Part model, mm, in its own coordinate system. Coordinates: 2 decimals unless noted, no trailing zeros. Order: outer loops, then holes, each group sorted by start corner. A loop starts at its lowest first (then second) coordinate and runs counter-clockwise, first axis right, second up.
1) Pin check, flat tips, straight feed: pin 1 Ø12 at (x, z) = (-60.5, 86) entering from -Y; pin 2 Ø6 at (y, z) = (-39.5, 130.5) entering from -X; pin 3 Ø1.5 at (y, z) = (-13.5, 134) entering from -X; pin 4 Ø10 at (x, z) = (-67.5, 26.5) entering from -Y. Stop position of each tip, or through.
2) Cut at C-C (y = -93.5). List the corners of the cut face in (x, z).
3) Cut at B-B (x = 14). List the corners of the cut face in (y, z), and give its area (3 significant figures).
4) Wall check: L1, parallel to Y at x = 12.5, z = 67; L2, parallel to Z at x = 67, y = -35; L3, parallel to X at y = -48, z = 54.5. Give the ranges that are in metal, low to high.
5) Cut at A-A (z = 69). List the corners of the cut face in (x, y).
```python
from build123d import *

# Parameters (mm, degrees)
BOSS_EXTRU_1_DEPTH            = 170
ENL_V_MAT_EXTRU_1_DEPTH       = 220
ENL_V_MAT_EXTRU_2_DEPTH       = 220
ENL_V_MAT_EXTRU_3_DEPTH       = 220
ENL_V_MAT_EXTRU_4_DEPTH       = 220
ENL_V_MAT_EXTRU_11_DEPTH      = 220
ENL_V_MAT_EXTRU_13_DEPTH      = 220
ENL_V_MAT_EXTRU_13_DEPTH_BACK = 220
ENL_V_MAT_EXTRU_14_DEPTH      = 220
ENL_V_MAT_EXTRU_15_DEPTH      = 220
ENL_V_MAT_EXTRU_15_DEPTH_BACK = 220
ENL_V_MAT_EXTRU_16_DEPTH      = 220
ENL_V_MAT_EXTRU_17_DEPTH      = 220
ENL_V_MAT_EXTRU_17_DEPTH_BACK = 220
ENL_V_MAT_EXTRU_18_DEPTH      = 220
ENL_V_MAT_EXTRU_19_DEPTH      = 220
ENL_V_MAT_EXTRU_19_DEPTH_BACK = 220
ENL_V_MAT_EXTRU_20_DEPTH      = 220
ENL_V_MAT_EXTRU_20_DEPTH_BACK = 220
ENL_V_MAT_EXTRU_21_DEPTH      = 220
ENL_V_MAT_EXTRU_21_DEPTH_BACK = 220
ENL_V_MAT_EXTRU_22_DEPTH      = 220
ENL_V_MAT_EXTRU_22_DEPTH_BACK = 220
ENL_V_MAT_EXTRU_23_DEPTH      = 220
ENL_V_MAT_EXTRU_23_DEPTH_BACK = 220
CONG_2_R                      = 15
ESQUISSE26_R                  = 11.42194069
BOSS_EXTRU_2_DEPTH            = 30
CONG_6_R                      = 10


with BuildPart() as part:
    # Esquisse1 → Boss.-Extru.1 (new body)
    with BuildSketch(Plane.XY):
        Polygon((-32, 85), (32, 85), (85, 32), (85, -32), (32, -85), (-32, -85), (-85, -32), (-85, 32), align=None)
    extrude(amount=BOSS_EXTRU_1_DEPTH)

    # Esquisse3D3 → Enlèv. mat.-Extru.1 (cut, along a direction that is not the sketch's normal)
    with BuildSketch(Plane(origin=(-32, 85, 117), x_dir=(0.6493531093113899, -0.5377455436484948, 0.5377455436484945), z_dir=(0, 0.7071067811865474, 0.7071067811865478))):
        Polygon((0, 0), (57.001027627, -48.67117062), (98.559626623, 0), (41.558598996, 48.67117062), align=None)
    extrude(amount=ENL_V_MAT_EXTRU_1_DEPTH, dir=(0, 0, 1), mode=Mode.SUBTRACT)

    # Esquisse3D4 → Enlèv. mat.-Extru.2 (cut, along a direction that is not the sketch's normal)
    with BuildSketch(Plane(origin=(32, 85, 53), x_dir=(-0.6493531093113893, -0.537745543648495, -0.537745543648495), z_dir=(0, -0.7071067811865476, 0.7071067811865476))):
        Polygon((0, 0), (57.001027627, 48.67117062), (98.559626623, 0), (41.558598996, -48.67117062), align=None)
    extrude(amount=-ENL_V_MAT_EXTRU_2_DEPTH, dir=(0, 0, 1), mode=Mode.SUBTRACT)

    # Esquisse3D5 → Enlèv. mat.-Extru.3 (cut, along a direction that is not the sketch's normal)
    with BuildSketch(Plane(origin=(-32, -85, 53), x_dir=(0.6493531093113899, 0.5377455436484946, -0.5377455436484948), z_dir=(0, 0.7071067811865479, 0.7071067811865472))):
        Polygon((0, 0), (57.001027627, 48.67117062), (98.559626623, 0), (41.558598996, -48.67117062), align=None)
    extrude(amount=-ENL_V_MAT_EXTRU_3_DEPTH, dir=(0, 0, 1), mode=Mode.SUBTRACT)

    # Esquisse3D6 → Enlèv. mat.-Extru.4 (cut, along a direction that is not the sketch's normal)
    with BuildSketch(Plane(origin=(32, -85, 117), x_dir=(-0.6493531093113899, 0.5377455436484946, 0.5377455436484947), z_dir=(0, 0.7071067811865476, -0.7071067811865476))):
        Polygon((0, 0), (57.001027627, 48.67117062), (98.559626623, 0), (41.558598996, -48.67117062), align=None)
    extrude(amount=-ENL_V_MAT_EXTRU_4_DEPTH, dir=(0, 0, -1), mode=Mode.SUBTRACT)

    # Esquisse3D13 → Enlèv. mat.-Extru.11 (cut, along a direction that is not the sketch's normal)
    with BuildSketch(Plane(origin=(32, 32, 170), x_dir=(0.5377455436484943, -0.6493531093113897, -0.5377455436484953), z_dir=(-0.7071067811865481, 0, -0.7071067811865469))):
        Polygon((0, 0), (57.001027627, -48.67117062), (98.559626623, 0), (41.558598996, 48.67117062), align=None)
    extrude(amount=-ENL_V_MAT_EXTRU_11_DEPTH, dir=(-1, 0, 0), mode=Mode.SUBTRACT)

    # Esquisse16 → Enlèv. mat.-Extru.13 (cut, two sides: drawn at the far end of the back side and taken through both)
    with BuildSketch(Plane(origin=(0, -32, 0), x_dir=(1, 0, 0), z_dir=(0, 1, 0)).offset(-ENL_V_MAT_EXTRU_13_DEPTH_BACK)):
        Polygon((32, -170), (85, -170), (85, -117), align=None)
    extrude(amount=ENL_V_MAT_EXTRU_13_DEPTH + ENL_V_MAT_EXTRU_13_DEPTH_BACK, mode=Mode.SUBTRACT)

    # Esquisse3D15 → Enlèv. mat.-Extru.14 (cut, along a direction that is not the sketch's normal)
    with BuildSketch(Plane(origin=(-85, -32, 117), x_dir=(0.5377455436484945, 0.6493531093113897, 0.5377455436484953), z_dir=(0.707106781186548, 0, -0.707106781186547))):
        Polygon((0, 0), (57.001027627, 48.67117062), (98.559626623, 0), (41.558598996, -48.67117062), align=None)
    extrude(amount=-ENL_V_MAT_EXTRU_14_DEPTH, dir=(0, 0, -1), mode=Mode.SUBTRACT)

    # Esquisse17 → Enlèv. mat.-Extru.15 (cut, two sides: drawn at the far end of the back side and taken through both)
    with BuildSketch(Plane(origin=(0, -32, 0), x_dir=(1, 0, 0), z_dir=(0, 1, 0)).offset(-ENL_V_MAT_EXTRU_15_DEPTH_BACK)):
        Polygon((-85, -117), (-32, -170), (-85, -170), align=None)
    extrude(amount=ENL_V_MAT_EXTRU_15_DEPTH + ENL_V_MAT_EXTRU_15_DEPTH_BACK, mode=Mode.SUBTRACT)

    # Esquisse3D16 → Enlèv. mat.-Extru.16 (cut, along a direction that is not the sketch's normal)
    with BuildSketch(Plane(origin=(-32, 32, 0), x_dir=(-0.5377455436484945, -0.6493531093113896, 0.5377455436484951), z_dir=(0.7071067811865479, 0, 0.7071067811865471))):
        Polygon((0, 0), (57.001027627, -48.67117062), (98.559626623, 0), (41.558598996, 48.67117062), align=None)
    extrude(amount=-ENL_V_MAT_EXTRU_16_DEPTH, dir=(0, 0, 1), mode=Mode.SUBTRACT)

    # Esquisse18 → Enlèv. mat.-Extru.17 (cut, two sides: drawn at the far end of the back side and taken through both)
    with BuildSketch(Plane(origin=(0, -32, 0), x_dir=(1, 0, 0), z_dir=(0, 1, 0)).offset(-ENL_V_MAT_EXTRU_17_DEPTH_BACK)):
        Polygon((-32, 0), (-85, -53), (-85, 0), align=None)
    extrude(amount=ENL_V_MAT_EXTRU_17_DEPTH + ENL_V_MAT_EXTRU_17_DEPTH_BACK, mode=Mode.SUBTRACT)

    # Esquisse3D17 → Enlèv. mat.-Extru.18 (cut, along a direction that is not the sketch's normal)
    with BuildSketch(Plane(origin=(85, 32, 53), x_dir=(-0.5377455436484941, -0.6493531093113903, -0.5377455436484949), z_dir=(0.707106781186548, 0, -0.707106781186547))):
        Polygon((0, 0), (57.001027627, 48.67117062), (98.559626623, 0), (41.558598996, -48.67117062), align=None)
    extrude(amount=ENL_V_MAT_EXTRU_18_DEPTH, dir=(0, 0, -1), mode=Mode.SUBTRACT)

    # Esquisse19 → Enlèv. mat.-Extru.19 (cut, two sides: drawn at the far end of the back side and taken through both)
    with BuildSketch(Plane(origin=(0, -32, 0), x_dir=(1, 0, 0), z_dir=(0, 1, 0)).offset(-ENL_V_MAT_EXTRU_19_DEPTH_BACK)):
        Polygon((85, -53), (32, 0), (85, 0), align=None)
    extrude(amount=ENL_V_MAT_EXTRU_19_DEPTH + ENL_V_MAT_EXTRU_19_DEPTH_BACK, mode=Mode.SUBTRACT)

    # Esquisse21 → Enlèv. mat.-Extru.20 (cut, two sides: drawn at the far end of the back side and taken through both)
    with BuildSketch(Plane.ZY.offset(-32).offset(-ENL_V_MAT_EXTRU_20_DEPTH_BACK)):
        Polygon((117, 85), (170, 32), (170, 85), align=None)
    extrude(amount=ENL_V_MAT_EXTRU_20_DEPTH + ENL_V_MAT_EXTRU_20_DEPTH_BACK, mode=Mode.SUBTRACT)

    # Esquisse23 → Enlèv. mat.-Extru.21 (cut, two sides: drawn at the far end of the back side and taken through both)
    with BuildSketch(Plane.ZY.offset(-32).offset(-ENL_V_MAT_EXTRU_21_DEPTH_BACK)):
        Polygon((0, 32), (53, 85), (0, 85), align=None)
    extrude(amount=ENL_V_MAT_EXTRU_21_DEPTH + ENL_V_MAT_EXTRU_21_DEPTH_BACK, mode=Mode.SUBTRACT)

    # Esquisse24 → Enlèv. mat.-Extru.22 (cut, two sides: drawn at the far end of the back side and taken through both)
    with BuildSketch(Plane.ZY.offset(-32).offset(-ENL_V_MAT_EXTRU_22_DEPTH_BACK)):
        Polygon((0, -32), (53, -85), (0, -85), align=None)
    extrude(amount=ENL_V_MAT_EXTRU_22_DEPTH + ENL_V_MAT_EXTRU_22_DEPTH_BACK, mode=Mode.SUBTRACT)

    # Esquisse25 → Enlèv. mat.-Extru.23 (cut, two sides: drawn at the far end of the back side and taken through both)
    with BuildSketch(Plane(origin=(-32, 0, 0), x_dir=(0, 0, -1), z_dir=(1, 0, 0)).offset(-ENL_V_MAT_EXTRU_23_DEPTH_BACK)):
        Polygon((-170, -32), (-170, -85), (-117, -85), align=None)
    extrude(amount=ENL_V_MAT_EXTRU_23_DEPTH + ENL_V_MAT_EXTRU_23_DEPTH_BACK, mode=Mode.SUBTRACT)

    # Congé2
    cong_2_edges = [part.edges().sort_by_distance(p)[0] for p in [
        (85, 32, 85),
        (85, -32, 85),
        (32, 0, 170),
        (85, 0, 117),
        (71.75, 45.25, 130.25),
        (-85, -32, 85),
        (-85, 32, 85),
        (-32, 0, 170),
        (-85, 0, 117),
        (-71.75, -45.25, 130.25),
        (-32, 0, 0),
        (-85, 0, 53),
        (-71.75, 45.25, 39.75),
        (85, 0, 53),
        (32, 0, 0),
        (71.75, -45.25, 39.75),
        (-71.75, 45.25, 130.25),
        (-45.25, 45.25, 156.75),
        (-32, 85, 85),
        (45.25, 45.25, 156.75),
        (45.25, 71.75, 130.25),
        (-45.25, 71.75, 130.25),
        (32, 85, 85),
        (71.75, 45.25, 39.75),
        (45.25, 45.25, 13.25),
        (-45.25, 45.25, 13.25),
        (-45.25, 71.75, 39.75),
        (45.25, 71.75, 39.75),
        (-71.75, -45.25, 39.75),
        (0, 32, 170),
        (-45.25, -71.75, 39.75),
        (-45.25, -45.25, 13.25),
        (45.25, -71.75, 39.75),
        (45.25, -45.25, 13.25),
        (0, 85, 117),
        (71.75, -45.25, 130.25),
        (-45.25, -45.25, 156.75),
        (-45.25, -71.75, 130.25),
        (45.25, -45.25, 156.75),
        (45.25, -71.75, 130.25),
        (0, 85, 53),
        (0, 32, 0),
        (0, -85, 53),
        (0, -32, 0),
        (32, -85, 85),
        (-32, -85, 85),
        (0, -32, 170),
        (0, -85, 117),
    ]]
    fillet(cong_2_edges, radius=CONG_2_R)

    # Esquisse26 → Boss.-Extru.2 (add)
    with BuildSketch(Plane.XZ.offset(85)):
        with Locations(Location((0, 85, 0), (0, 0, 180))):
            Circle(ESQUISSE26_R)
    extrude(amount=BOSS_EXTRU_2_DEPTH)

    # Congé6
    cong_6_edges = [part.edges().sort_by_distance(p)[0] for p in [
        (11.42194069, -115, 85),
    ]]
    fillet(cong_6_edges, radius=CONG_6_R)


solid = part.part
```
Geometry check:
1. pin 1: stops at y = -62.5
1. pin 2: stops at x = -73.22
1. pin 3: stops at x = -68.75
1. pin 4: passes through
2. outline: circle Ø22.84 at (0, 85)
3. outline: (-85, 59.21) arc R15 ccw to (-80.61, 48.61) - (-36.39, 4.39) arc R15 ccw to (-25.79, 0) - (25.79, 0) arc R15 ccw to (36.39, 4.39) - (80.61, 48.61) arc R15 ccw to (85, 59.21) - (85, 110.79) arc R15 ccw to (80.61, 121.39) - (36.39, 165.61) arc R15 ccw to (25.79, 170) - (-25.79, 170) arc R15 ccw to (-36.39, 165.61) - (-80.61, 121.39) arc R15 ccw to (-85, 110.79) - close
3. area: 23,200 mm2
4. L1: y = -85 to 85
4. L2: z = 35 to 135
4. L3: x = -69 to 69
5. outline: (-85, -25.79) arc R15 ccw to (-80.61, -36.39) - (-36.39, -80.61) arc R15 ccw to (-25.79, -85) - (25.79, -85) arc R15 ccw to (36.39, -80.61) - (80.61, -36.39) arc R15 ccw to (85, -25.79) - (85, 25.79) arc R15 ccw to (80.61, 36.39) - (36.39, 80.61) arc R15 ccw to (25.79, 85) - (-25.79, 85) arc R15 ccw to (-36.39, 80.61) - (-80.61, 36.39) arc R15 ccw to (-85, 25.79) - close
